```python
from build123d import *

# Parameters (mm, degrees)
SKETCH_1_R      = 2.4
EXTRUDE_1_DEPTH = 40
SKETCH_2_R      = 2.5
EXTRUDE_2_DEPTH = 10
SKETCH_3_R      = 11
SKETCH_3_R_2    = 1.5
SKETCH_3_R_3    = 2.4
EXTRUDE_3_DEPTH = 2


with BuildPart() as part:
    # Sketch 1 → Extrude 1 (new body)
    with BuildSketch(Plane(origin=(0, 0, 0), x_dir=(1, 0, 0), z_dir=(0, 1, 0))):
        with Locations(Location((0, 0, 0), (0, 0, 270))):
            Circle(SKETCH_1_R)
    extrude(amount=EXTRUDE_1_DEPTH)

    # Sketch 2 → Extrude 2 (add, symmetric)
    with BuildSketch(Plane(origin=(0, 20, 0), x_dir=(-1, 0, 0), z_dir=(0, -1, 0))):
        with Locations(Location((0, 0, 0), (0, 0, 90))):
            Circle(SKETCH_2_R)
    extrude(amount=EXTRUDE_2_DEPTH, both=True)



with BuildPart() as body_2:
    # Sketch 3 → Extrude 3 (new body)
    with BuildSketch(Plane.XZ):
        with Locations(Location((0, 0, 0), (0, 0, 270))):
            Circle(SKETCH_3_R)
        with Locations(Location((-5, -5, 0), (0, 0, 270))):
            Circle(SKETCH_3_R_2, mode=Mode.SUBTRACT)
        with Locations(Location((-5, 5, 0), (0, 0, 270))):
            Circle(SKETCH_3_R_2, mode=Mode.SUBTRACT)
        with Locations(Location((5, 5, 0), (0, 0, 270))):
            Circle(SKETCH_3_R_2, mode=Mode.SUBTRACT)
        with Locations(Location((5, -5, 0), (0, 0, 270))):
            Circle(SKETCH_3_R_2, mode=Mode.SUBTRACT)
        with Locations(Location((0, 0, 0), (0, 0, 270))):
            Circle(SKETCH_3_R_3, mode=Mode.SUBTRACT)
    extrude(amount=EXTRUDE_3_DEPTH)


with BuildPart() as part_1:
    add(part.part)

    add(body_2.part)  # Revolve 3 merges body 2
    # Sketch 4 → Revolve 3 (revolve)
    with BuildSketch(Plane(origin=(0, 0, 0), x_dir=(0, 0, -1), z_dir=(1, 0, 0)), mode=Mode.PRIVATE) as revolve_3_sk:
        with BuildLine():
            Line((-2.4, 0), (-4.4, 0))
            ThreePointArc((-4.4, 0), (-2.985786438, 0.585786438), (-2.4, 2))
            Line((-2.4, 2), (-2.4, 0))
        make_face()
    revolve(revolve_3_sk.sketch.rotate(Axis((0, -1000, 0), (0, 1, 0)), 180), axis=Axis((0, -1000, 0), (0, 1, 0)))


solid = part_1.part
```
Geometry: final body of the model. Coordinates: model frame, mm. A direction names the side the tool comes from. Coordinates: 2 decimals unless noted, no trailing zeros. Write each loop counter-clockwise with the first axis right and the second up, starting at its lowest first coordinate (ties: lowest second). Pieces come first, ordered by that corner, then holes. Notation, with made-up numbers: M 38,-0.75 L 50,-0.75 A27 cw 50,32.25 Z; hole C 29,22 d1. An arc over 180 degrees is marked long. Use CSV: the item, a comma, the result in double quotes. Start each with the question number.
1. First-contact query: P1, Ø3.5, axis at x = -5, z = 5, coming from the +Y side; P2, Ø1.4, axis at x = 1, z = -0.5, coming from the -Y side; P3, Ø3, axis at y = 21, z = -1, coming from the -X side. Flat tips, straight axial feed; report the tip coordinate or a pass-through.
2. Cut plane B-B on x = -5. Return the cut outline in (y, z), plus the area to 3 significant figures.
3. Cut plane C-C on x = 0. Return the cut outline in (y, z), plus the area to 3 significant figures.
4. Reachability of faces 1 (the face through (-5, 0, 0)), 2 (the face through (2.024, -0.986, -1.29)), 3 (the face through (-4.55, -0.99, -6.43)) from +Z, -Z, +X, -X, +Y, -Y: full face, straight path, thin tool, end or side. Return the list, or none.
5. Mould query, pull axis Y, two halves, no side actions, for faces 4 (the face through (0, 0, 0)), 5 (the face through (2.024, 5.944, 1.29)), 6 (the face through (0, 40, 0)), 7 (the face through (-3.99, -0.99, 6.11)). Classes: pulls with the +Y half, pulls with the -Y half, needs draft (parallel to the pull), parting line crosses it, or undercut.
6. Cut plane A-A on z = 0. Return the cut outline in (x, y), plus the area to 3 significant figures.
7. Ray query, probe 1 along X at (y, z) = (-1.5, -5); probe 2 along Y at (x, z) = (-7.5, -1); probe 3 along Z at (x, y) = (-2, 23). Return the intervals inside material, ascending.
8. Cut plane D-D on z = -5. Return the cut outline in (x, y).
Entries:
1,P1,"y = 0"
1,P2,"y = 0"
1,P3,"x = -2.5"
2,outline,"M -2,-9.8 L 0,-9.8 L 0,-6.5 L -2,-6.5 Z; M -2,-3.5 L 0,-3.5 L 0,3.5 L -2,3.5 Z; M -2,6.5 L 0,6.5 L 0,9.8 L -2,9.8 Z"
2,area,"27.2 mm²"
3,outline,"M -2,-11 L 0,-11 L 0,-4.4 A2 cw 2,-2.4 L 10,-2.4 L 10,-2.5 L 30,-2.5 L 30,-2.4 L 40,-2.4 L 40,2.4 L 30,2.4 L 30,2.5 L 10,2.5 L 10,2.4 L 2,2.4 A2 cw 0,4.4 L 0,11 L -2,11 L -2,2.4 L 0,2.4 L 0,-2.4 L -2,-2.4 Z"
3,area,"232 mm²"
4,face 1,"+Y"
4,face 2,"-Y"
4,face 3,"+Y, -Y"
5,face 4,"pulls with the -Y half"
5,face 5,"undercut"
5,face 6,"pulls with the +Y half"
5,face 7,"needs draft"
6,outline,"M -11,-2 L -2.4,-2 L -2.4,0 L 2.4,0 L 2.4,-2 L 11,-2 L 11,0 L 4.4,0 A2 cw 2.4,2 L 2.4,10 L 2.5,10 L 2.5,30 L 2.4,30 L 2.4,40 L -2.4,40 L -2.4,30 L -2.5,30 L -2.5,10 L -2.4,10 L -2.4,2 A2 cw -4.4,0 L -11,0 Z"
6,area,"232 mm²"
7,probe 1,"-9.8 to -6.5, -3.5 to 3.5, 6.5 to 9.8"
7,probe 2,"-2 to 0"
7,probe 3,"-1.5 to 1.5"
8,outline,"M -9.8,-2 L -6.5,-2 L -6.5,0 L -9.8,0 Z; M -3.5,-2 L 3.5,-2 L 3.5,0 L -3.5,0 Z; M 6.5,-2 L 9.8,-2 L 9.8,0 L 6.5,0 Z"
